The listing builds one solid part. Answer for the finished solid, in the listing's coordinates (mm). A direction names the side the tool comes from. Coordinates: 2 decimals unless noted, no trailing zeros. Order: outer loops, then holes, each group sorted by start corner. A loop starts at its lowest first (then second) coordinate and runs counter-clockwise, first axis right, second up. Notation, with made-up numbers: (61, 58.5) -> (82, 58.5) arc R17 cw to (82, 85.5) -> close; hole circle Ø3 at (62.5, 86). An arc over 180 degrees is marked (long way). One line per question, with ' | ' between items.
from build123d import *

# Parameters (mm, degrees)
F1_DEPTH     = 12
F2_W         = 5.9
F2_H         = 13.7
F3_DEPTH     = 12.001
F4_R         = 1.6
F5_DEPTH     = 20.001
F6_R         = 0.95
F7_DEPTH     = 7
F9_DEPTH     = 4
F10_R        = 2.8
F11_DEPTH    = 3
F12_T1_DEPTH = 37


# Not quite as in the source:
# - a fillet or chamfer that OpenCascade refuses, or shapes differently, is made with other operations: its cross-section is extruded or revolved along the edge and cut away or added


with BuildPart() as f1:
    # F0 (on Top) → F1 (new body)
    with BuildSketch(Plane.XY):
        with BuildLine():
            Line((18, 10), (-16, 10))
            Line((-16, 10), (-16, 1))
            Line((-16, 1), (-5.0009999, 1))
            ThreePointArc((-5.0009999, 1), (5.1, 0), (-5.0009999, -1))
            Line((-5.0009999, -1), (-16, -1))
            Line((-16, -1), (-16, -10))
            Line((-16, -10), (18, -10))
            Line((18, -10), (18, -6.85))
            Line((18, -6.85), (18, 6.85))
            Line((18, 6.85), (18, 10))
        make_face()
    extrude(amount=F1_DEPTH)

    # F2 (on face) → F3 (cut, through all)
    with BuildSketch(Plane(origin=(0, 0, 0), x_dir=(1, 0, 0), z_dir=(0, 0, -1))):
        with Locations((15.05, 0)):
            Rectangle(F2_W, F2_H)
    extrude(amount=-F3_DEPTH, mode=Mode.SUBTRACT)

    # F4 (on face) → F5 (cut, through all)
    with BuildSketch(Plane.XZ.offset(10)):
        with Locations((-10.3, 6)):
            Circle(F4_R)
    extrude(amount=-F5_DEPTH, mode=Mode.SUBTRACT)

    # F6 (on face) → F7 (cut)
    with BuildSketch(Plane.YZ.offset(12.1)):
        with Locations((-3.25, 5)):
            Circle(F6_R)
        with Locations((3.25, 5)):
            Circle(F6_R)
    extrude(amount=-F7_DEPTH, mode=Mode.SUBTRACT)

    # F8 (on face) → F9 (cut)
    with BuildSketch(Plane.XZ.offset(10)):
        Polygon((-7.5270084947, 4.4889189478), (-7.5736076532, 7.5934053818), (-10.3445898285, 8.994), (-13.0481386516, 7.4672939832), (-13.0481386516, 4.3624578361), (-10.2550660504, 3.006451588), align=None)
    extrude(amount=-F9_DEPTH, mode=Mode.SUBTRACT)

    # F10 (on face) → F11 (cut)
    with BuildSketch(Plane(origin=(0, 10, 0), x_dir=(-1, 0, 0), z_dir=(0, 1, 0))):
        with Locations((10.3, 6)):
            Circle(F10_R)
    extrude(amount=-F11_DEPTH, mode=Mode.SUBTRACT)

    # F12: fillet of radius 5 on 2 edges, made by hand

    # F12_s2 → F12_t1 (cut)
    with BuildSketch(Plane.XY.offset(-12.5)):
        with BuildLine():
            ThreePointArc((-11, -10), (-14.5355339059, -8.5355339059), (-16, -5))
            Line((-16, -5), (-16, -10))
            Line((-16, -10), (-11, -10))
        make_face()
        with BuildLine():
            ThreePointArc((-16, 5), (-14.5355339059, 8.5355339059), (-11, 10))
            Line((-11, 10), (-16, 10))
            Line((-16, 10), (-16, 5))
        make_face()
    extrude(amount=F12_T1_DEPTH, mode=Mode.SUBTRACT)


solid = f1.part
Item 1: For faces 4 (the face through (5.1, -3, 5)), 5 (the face through (-9.1, -6, 4.7)), 6 (the face through (15, -6.85, 6)), 7 (the face through (-9.2, -1, 4.6)), 8 (the face through (-12, 7, 5)), determine the directions among +Z, -Z, +X, -X, +Y, -Y from which every point of the face is accessible in a straight line to the end or side of a thin tool.
Computed values:
face 4: +X | face 5: -Y | face 6: +Z, -Z, +X | face 7: +Z, -Z, -X | face 8: +Y
Item 2: Each of these flat-tipped pins is pushed along its axis until it touches: pin 1 Ø2.5 at (x, z) = (-10.3, 6) entering from +Y; pin 2 Ø3.5 at (x, z) = (-10.3, 6) entering from +Y; pin 3 Ø6 at (y, z) = (1, 6.5) entering from +X. Where does it stop, or does it pass through?
Computed values:
pin 1: passes through | pin 2: stops at y = 7 | pin 3: stops at x = 12.1
Item 3: Section B-B, the plane y = -3.75 is taken. Give the vertices of the cut face in (x, z), plus the area to 3 significant figures.
Computed values:
outline: (-16, 0) -> (-3.46, 0) -> (-3.46, 12) -> (-16, 12) -> close; (3.46, 0) -> (12.1, 0) -> (12.1, 4.19) -> (5.1, 4.19) -> (5.1, 5.81) -> (12.1, 5.81) -> (12.1, 12) -> (3.46, 12) -> close; hole circle Ø3.2 at (-10.3, 6) | area: 235 mm^2
Item 4: Section C-C, the plane z = 6.5 is taken. Give the vertices of the cut face in (x, y) (3 decimals), plus the area to 3 significant figures.
Computed values:
outline: (-16, -5) arc R5 ccw to (-13.048, -9.561) -> (-13.048, -6) -> (-11.82, -6) -> (-11.82, -1) -> (-16, -1) -> close; (-16, 1) -> (-11.82, 1) -> (-11.82, 7) -> (-13.055, 7) -> (-13.055, 9.558) arc R5 ccw to (-16, 5) -> close; (-8.78, -6) -> (-7.557, -6) -> (-7.557, -10) -> (18, -10) -> (18, -6.85) -> (12.1, -6.85) -> (12.1, 6.85) -> (18, 6.85) -> (18, 10) -> (-7.545, 10) -> (-7.545, 7) -> (-8.78, 7) -> (-8.78, 1) -> (-5.001, 1) arc R5.1 cw (long way) to (-5.001, -1) -> (-8.78, -1) -> close | area: 414 mm^2
Item 5: Section A-A, the plane x = 13 is taken. Give the vertices of the cut face in (y, z).
Computed values:
outline: (-10, 0) -> (-6.85, 0) -> (-6.85, 12) -> (-10, 12) -> close; (6.85, 0) -> (10, 0) -> (10, 12) -> (6.85, 12) -> close
Item 6: Determine the mould class of faces 1 (the face through (3, -10, 6)), 2 (the face through (-11.68, -8.03, 8.24)), 3 (the face through (-12, 1, 5)) for opening direction Y: pulls with the +Y half, pulls with the -Y half, needs draft (parallel to the pull), parting line crosses it, or undercut.
Computed values:
face 1: pulls with the -Y half | face 2: needs draft | face 3: undercut
Item 7: Section D-D, the plane x = -11.5 is taken. Give the vertices of the cut face in (y, z).
Computed values:
outline: (-9.97, 0) -> (-1, 0) -> (-1, 4.94) -> (-6, 4.94) -> (-6, 3.61) -> (-9.97, 3.61) -> close; (-9.97, 8.34) -> (-6, 8.34) -> (-6, 7.06) -> (-1, 7.06) -> (-1, 12) -> (-9.97, 12) -> close; (1, 0) -> (9.97, 0) -> (9.97, 3.47) -> (7, 3.47) -> (7, 4.94) -> (1, 4.94) -> close; (1, 7.06) -> (7, 7.06) -> (7, 8.53) -> (9.97, 8.53) -> (9.97, 12) -> (1, 12) -> close
Item 8: Find the intervals of material crossed by L1, parallel to Y at x = -9.5, z = 10.75; L2, parallel to Y at x = 15.5, z = 11; L3, parallel to Z at x = 9, y = -3.25, in increasing order.
Computed values:
L1: y = -10 to -1, 1 to 10 | L2: y = -10 to -6.85, 6.85 to 10 | L3: z = 0 to 4.05, 5.95 to 12
